Autodesk Inventor part; units mm, degrees
ref_plane "YZ Plane" through (0, 0, 0) normal (1, 0, 0) x (0, 1, 0)
ref_plane "XZ Plane" through (0, 0, 0) normal (0, 1, 0) x (-1, 0, 0)
ref_plane "XY Plane" through (0, 0, 0) normal (0, 0, 1) x (1, 0, 0)
sketch "Sketch1" plane through (0, 0, 0) normal (0, 1, 0) x (-1, 0, 0)
  line L0 (190, -125) -> (-190, -125)
  line L1 (-190, -125) -> (-190, 125)
  line L2 (-190, 125) -> (190, 125)
  line L3 (190, 125) -> (190, -125)
  line L4 (190, -125) -> (-190, 125) construction
  line L5 (-190, -125) -> (190, 125) construction
  line L6 (-60, 75) -> (60, 75) construction
  line L7 (60, 75) -> (60, -75) construction
  line L8 (60, -75) -> (-60, -75) construction
  line L9 (-60, -75) -> (-60, 75) construction
  line L10 (-60, 75) -> (60, -75) construction
  line L11 (60, 75) -> (-60, -75) construction
  line L12 (-156, 125) -> (156, 125)
  line L13 (156, 125) -> (156, -125)
  line L14 (156, -125) -> (-156, -125)
  line L15 (-156, -125) -> (-156, 125)
  line L16 (-156, 125) -> (156, -125) construction
  line L17 (156, 125) -> (-156, -125) construction
  point P0 (0, 0)
  dimension "d0" = 380
  dimension "d1" = 250
  dimension "d2" = 120
  dimension "d3" = 150
  dimension "d16" = 312
extrude "Extrusion1" add sketch "Sketch1" along normal blind 40
hole "Hole1" at (-60, 0, -75) at (60, 0, -75) at (60, 0, 75) at (-60, 0, 75) direction (0, 1, 0) diameter 8 end through all
sketch "Sketch2" plane through (-190, 0, 125) normal (0, 0, 1) x (1, 0, 0)
  line L0 (0, 0) -> (380, 0) construction
  line L1 (0, 40) -> (380, 40) construction
  line L2 (380, 0) -> (0, 40) construction
  line L3 (0, 0) -> (380, 40) construction
  circle A0 centre (190, 20) radius 15
  point P0 (190, 0)
  dimension "d13" = 30
extrude "Extrusion2" cut sketch "Sketch2" against normal through all
extrude "Extrusion3" add sketch "Sketch1" along normal blind 120 contours L0 L13 L2 L3 | L0 L1 L2 L15
sketch "Sketch3" plane through (-190, 0, -125) normal (-1, 0, 0) x (0, 0, 1)
  line L0 (170, 97.5) -> (220, 97.5) construction
  line L1 (220, 97.5) -> (220, 62.5) construction
  line L2 (220, 62.5) -> (170, 62.5) construction
  line L3 (170, 62.5) -> (170, 97.5) construction
  line L4 (170, 97.5) -> (220, 62.5) construction
  line L5 (220, 97.5) -> (170, 62.5) construction
  line L6 (0, 0) -> (250, 0) construction
  line L7 (125, 0) -> (125, 120) construction
  line L8 (0, 120) -> (250, 120) construction
  line L9 (80, 97.5) -> (30, 97.5) construction
  line L10 (30, 97.5) -> (30, 62.5) construction
  line L11 (30, 62.5) -> (80, 62.5) construction
  line L12 (80, 62.5) -> (80, 97.5) construction
  line L13 (80, 97.5) -> (30, 62.5) construction
  line L14 (30, 97.5) -> (80, 62.5) construction
  point P0 (195, 80)
  point P1 (55, 80)
  dimension "d19" = 50
  dimension "d20" = 35
  dimension "d21" = 62.5
  dimension "d22" = 70
hole "Hole2" at (-190, 97.5, 45) at (-190, 97.5, 95) at (-190, 62.5, 95) at (-190, 62.5, 45) at (-190, 62.5, -45) at (-190, 62.5, -95) at (-190, 97.5, -95) at (-190, 97.5, -45) direction (1, 0, 0) diameter 8 end through all
chamfer "Chamfer1" distance 5 angle 45 10 edges at (-190, 120, 0) (-173, 120, 125) (-156, 120, 0) (-173, 120, -125) (156, 120, 0) (190, 120, 0) (173, 120, -125) (173, 120, 125) (-190, 0, 0) (190, 0, 0)
properties part number "SACMI DPA TILES GRIP FIXED SUPPORT"
Check sheet for the modelled part. Datum: model origin and axes. Units: mm. A direction names the side the tool comes from. Round coordinates to 2 decimals unless told otherwise and drop trailing zeros. Loops run counter-clockwise (first coordinate to the right, second up) from the corner with the lowest first, then second, coordinate; pieces in that order, holes last. Notation, with made-up numbers: (70.5, -31) -> (80.5, -31) arc R23 cw to (80.5, -1) -> close; hole circle Ø6 at (1.25, -32.75). An arc over 180 degrees is marked (long way). Answer in a Markdown table with one row per item.
Q1. Sectioned sample at D-D on z = 75. Enter the section's corners in (x, y).
Data:
| item | result |
|---|---|
| outline | (-190, 5) -> (-185, 0) -> (-64, 0) -> (-64, 40) -> (-156, 40) -> (-156, 115) -> (-161, 120) -> (-185, 120) -> (-190, 115) -> close; (-56, 0) -> (56, 0) -> (56, 40) -> (-56, 40) -> close; (64, 0) -> (185, 0) -> (190, 5) -> (190, 115) -> (185, 120) -> (161, 120) -> (156, 115) -> (156, 40) -> (64, 40) -> close; hole circle Ø30 at (0, 20) |
Q2. Thickness scan on L1, parallel to Z at x = -170, y = 97; L2, parallel to Z at x = 60, y = 21; L3, parallel to Y at x = -175, z = 95. Record the ranges inside material, lowest first.
Data:
| item | result |
|---|---|
| L1 | z = -125 to -98.97, -91.03 to -48.97, -41.03 to 41.03, 48.97 to 91.03, 98.97 to 125 |
| L2 | z = -125 to -79, -71 to 71, 79 to 125 |
| L3 | y = 0 to 58.5, 66.5 to 93.5, 101.5 to 120 |
Q3. Release check for a two-part mould opening along Z. For faces 3 (the face through (-172.762, 66.405, 44.133)), 4 (the face through (-3.252, 5.357, 1.75)) record: released by +Z, released by -Z, zero draft, split by the parting line, or undercut.
Data:
| item | result |
|---|---|
| face 3 | undercut |
| face 4 | zero draft |
Q4. Sectioned sample at B-B on y = 20. Enter the section's corners in (x, z).
Data:
| item | result |
|---|---|
| outline | (-190, -125) -> (-15, -125) -> (-15, 125) -> (-190, 125) -> close; (15, -125) -> (190, -125) -> (190, 125) -> (15, 125) -> close; hole circle Ø8 at (-60, -75); hole circle Ø8 at (-60, 75); hole circle Ø8 at (60, -75); hole circle Ø8 at (60, 75) |
Q5. Sectioned sample at C-C on x = 0. Enter the section's corners in (y, z).
Data:
| item | result |
|---|---|
| outline | (0, -125) -> (5, -125) -> (5, 125) -> (0, 125) -> close; (35, -125) -> (40, -125) -> (40, 125) -> (35, 125) -> close |
Q6. Go/stop test with flat-tipped pins: P1, Ø18, axis at x = 0, y = 20, coming from the -Z side; P2, Ø6, axis at x = 140, z = 31.5, coming from the +Y side. Record where each tip stops, or that it passes through.
Data:
| item | result |
|---|---|
| P1 | passes through |
| P2 | stops at y = 40 |
Q7. Set-up check for faces 1 (the face through (2, 40, 2)), 2 (the face through (173.238, 66.405, 44.133)): record each of +Z, -Z, +X, -X, +Y, -Y from which the full face is reachable in a straight line by a thin tool's end or side.
Data:
| item | result |
|---|---|
| face 1 | +Z, -Z, +Y |
| face 2 | +X, -X |
Q8. Sectioned sample at A-A on z = 45. Give the number of separate pieces and of enclosed holes in the cut face, then the cut area to 3 significant figures.
Data:
| item | result |
|---|---|
| separate pieces | 5 |
| enclosed holes | 1 |
| area | 18,800 mm^2 |
